Work out the finished part from the listing and answer in its coordinate system (mm). A direction names the side the tool comes from. Round coordinates to 2 decimals unless told otherwise and drop trailing zeros. Loops run counter-clockwise (first coordinate to the right, second up) from the corner with the lowest first, then second, coordinate; pieces in that order, holes last. Notation, with made-up numbers: (23, 26) -> (79, 26) arc R22 cw to (79, 60) -> close; hole circle Ø10 at (-14.75, -26). An arc over 180 degrees is marked (long way). Use one line per item in the form item = value.
```python
from build123d import *

# Parameters (mm, degrees)
BOSS_EXTRUDE1_DEPTH = 5.08


with BuildPart() as part:
    # Sketch1 → Boss-Extrude1 (new body)
    with BuildSketch(Plane.XY):
        with BuildLine():
            Line((149.742446498, 0.425166718), (142.412299482, 136.517741625))
            ThreePointArc((142.412299482, 136.517741625), (141.974063379, 138.670668966), (140.930746882, 140.604224682))
            ThreePointArc((140.930746882, 140.604224682), (135.996353851, 143.53718437), (130.433295393, 142.121957281))
            Line((130.433295393, 142.121957281), (69.876767595, 96.864174071))
            ThreePointArc((69.876767595, 96.864174071), (66.943807907, 91.92978104), (68.359034997, 86.366722582))
            Line((68.359034997, 86.366722582), (136.245709811, -4.468069115))
            ThreePointArc((136.245709811, -4.468069115), (139.075136314, -6.771534614), (142.656678242, -7.467354313))
            ThreePointArc((142.656678242, -7.467354313), (144.809605584, -7.02911821), (146.7431613, -5.985801713))
            ThreePointArc((146.7431613, -5.985801713), (149.046626799, -3.15637521), (149.742446498, 0.425166718))
        make_face()
        with BuildLine():
            ThreePointArc((72.989736811, 92.698910254), (76.208955267, 92.233472258), (75.74351727, 89.014253801))
            ThreePointArc((75.74351727, 89.014253801), (72.524298814, 89.479691798), (72.989736811, 92.698910254))
        make_face(mode=Mode.SUBTRACT)
        with BuildLine():
            Line((128.442984245, 116.978229985), (133.206299189, 28.541832403))
            ThreePointArc((133.206299189, 28.541832403), (132.371004795, 27.279573488), (130.920851777, 27.713244469))
            Line((130.920851777, 27.713244469), (86.384644261, 87.304278258))
            ThreePointArc((86.384644261, 87.304278258), (85.90535402, 89.188300722), (86.898649701, 90.859415162))
            Line((86.898649701, 90.859415162), (124.386094861, 118.87619102))
            ThreePointArc((124.386094861, 118.87619102), (126.982999322, 119.142292563), (128.442984245, 116.978229985))
        make_face(mode=Mode.SUBTRACT)
        with BuildLine():
            ThreePointArc((135.046856931, 133.817694213), (132.626483815, 135.990663145), (134.799452746, 138.411036261))
            ThreePointArc((134.799452746, 138.411036261), (137.219825863, 136.238067329), (135.046856931, 133.817694213))
        make_face(mode=Mode.SUBTRACT)
    extrude(amount=BOSS_EXTRUDE1_DEPTH)


solid = part.part
```
(1) For faces 4 (the flat face through (108.965, 57.092, 2.504)), 5 (the flat face through (135, 69, 5.08)), determine the directions among +Z, -Z, +X, -X, +Y, -Y from which every point of the face is accessible in a straight line to the end or side of a thin tool.
Completed:
face_4 = +Z, -Z
face_5 = +Z, +X, -X, +Y, -Y
(2) Given P1, Ø1, axis at x = 89.5, z = 1.5, coming from the -Y side, flat-ended and moving along its own axis, determine where the tip first touches the part or whether it passes through.
Completed:
P1 = 57.41
(3) For a pull along X with two mould halves and no side action, classify faces 1 (the flat face through (135, 69, 0)), 2 (the cylindrical face through (126.948, 119.158, 2.504)), 3 (the flat face through (101.827, 41.585, 2.504)) as +X half, -X half, draft (parallel to the pull), parting line (faces both ways), or undercut.
Completed:
face_1 = draft
face_2 = undercut
face_3 = -X half
(4) Find section C-C, the plane x = 98. Write down the section's boundary in (y, z).
Completed:
outline = (46.71, 0) -> (71.76, 0) -> (71.76, 5.08) -> (46.71, 5.08) -> close; (99.16, 0) -> (117.88, 0) -> (117.88, 5.08) -> (99.16, 5.08) -> close
(5) Find section D-D, the plane x = 144.5. Write down the section's boundary in (y, z), then the cut area to 3 significant figures.
Completed:
outline = (-7.13, 0) -> (97.76, 0) -> (97.76, 5.08) -> (-7.13, 5.08) -> close
area = 533 mm2
(6) Consider L1, parallel to Y at x = 101, z = 1.75; L2, parallel to X at y = 51.5, z = 2; L3, parallel to Y at x = 92.5, z = 2.2. Determine where each line is inside the solid, lowest interval first.
Completed:
L1 = 42.69 to 67.75, 101.4 to 120.12
L2 = 94.42 to 113.14, 131.97 to 146.99
L3 = 54.07 to 79.12, 95.05 to 113.77
(7) Find section B-B, the plane z = 1.9. Write down the section's boundary in (x, y), then the cut area to 3 significant figures.
Completed:
outline = (68.36, 86.37) -> (136.25, -4.47) arc R7.5 ccw to (149.74, 0.43) -> (142.41, 136.52) arc R7.5 ccw to (130.43, 142.12) -> (69.88, 96.86) arc R7.5 ccw to start; hole circle Ø4.6 at (74.37, 90.86); hole (86.38, 87.3) -> (130.92, 27.71) arc R1.27 ccw to (133.21, 28.54) -> (128.44, 116.98) arc R2.54 ccw to (124.39, 118.88) -> (86.9, 90.86) arc R2.54 ccw to start; hole circle Ø4.6 at (134.92, 136.11)
area = 4,690 mm2
(8) Find section A-A, the plane y = 71. Write down the section's boundary in (x, z).
Completed:
outline = (79.84, 0) -> (98.57, 0) -> (98.57, 5.08) -> (79.84, 5.08) -> close; (130.92, 0) -> (145.94, 0) -> (145.94, 5.08) -> (130.92, 5.08) -> close
